Could you check a few things on this model? Use its own coordinates, in mm. Face numbers are marked on the shaded views. A direction names the side the tool comes from. Give positions to 0.01 mm unless a question says otherwise; leave off trailing zeros. Loops run counter-clockwise (first coordinate to the right, second up) from the corner with the lowest first, then second, coordinate; pieces in that order, holes last. Notation, with made-up numbers: (-21, 45.5) -> (-4, 45.5) arc R19 ccw to (-4, 55.5) -> close; hole circle Ø7 at (-12.75, 16). An arc over 180 degrees is marked (long way). Put each result on its own line as item: value.
Autodesk Inventor part; units mm, degrees
ref_plane "YZ Plane" through (0, 0, 0) normal (1, 0, 0) x (0, 1, 0)
ref_plane "XZ Plane" through (0, 0, 0) normal (0, 1, 0) x (-1, 0, 0)
ref_plane "XY Plane" through (0, 0, 0) normal (0, 0, 1) x (1, 0, 0)
sketch "Sketch2" plane through (0, 0, 0) normal (0, 1, 0) x (-1, 0, 0)
  line L0 (18.3186, 20.469) -> (-22.6814, 20.469)
  line L1 (-22.6814, 20.469) -> (-22.6814, -20.531)
  line L2 (-22.6814, -20.531) -> (18.3186, -20.531)
  line L3 (18.3186, -20.531) -> (18.3186, 20.469)
  line L4 (-27.6814, 25.469) -> (23.3186, 25.469)
  line L5 (23.3186, 25.469) -> (23.3186, -25.531)
  line L6 (23.3186, -25.531) -> (-27.6814, -25.531)
  line L7 (-27.6814, -25.531) -> (-27.6814, 25.469)
  line L8 (-22.6814, 20.469) -> (18.3186, 20.469)
  line L9 (18.3186, 20.469) -> (18.3186, -20.531)
  line L10 (18.3186, -20.531) -> (-22.6814, -20.531)
  line L11 (-22.6814, -20.531) -> (-22.6814, 20.469)
  line L12 (-22.6814, 20.469) -> (18.3186, 20.469)
  line L13 (18.3186, 20.469) -> (18.3186, -20.531)
  line L14 (18.3186, -20.531) -> (-22.6814, -20.531)
  line L15 (-22.6814, -20.531) -> (-22.6814, 20.469)
  point P0 (0, 0)
  dimension "d0" = 41
  dimension "d1" = 41
  dimension "d6" = 5
extrude "Extrusion1" add sketch "Sketch2" along normal blind 10 contours L3 L2 L1 L0 | L4 L5 L6 L7
sketch "Sketch5" plane through (0, 0, 0) normal (0, -1, 0) x (1, 0, 0)
  line L0 (27.6814, 25.469) -> (-23.3186, 25.469)
  line L1 (-23.3186, 25.469) -> (-23.3186, -25.531)
  line L2 (-23.3186, -25.531) -> (27.6814, -25.531)
  line L3 (27.6814, -25.531) -> (27.6814, 25.469)
  line L4 (-18.3186, 20.469) -> (22.6814, 20.469)
  line L5 (22.6814, 20.469) -> (22.6814, -20.531)
  line L6 (22.6814, -20.531) -> (-18.3186, -20.531)
  line L7 (-18.3186, -20.531) -> (-18.3186, 20.469)
  point P0 (0, 0)
  dimension "d10" = 5
extrude "Extrusion2" cut sketch "Sketch5" against normal blind 4 contours L4 L5 L6 L7
fillet "Fillet1" radius 3 4 edges at (-23.3186, 10, -0.031) (2.1814, 10, 25.469) (27.6814, 10, -0.031) (2.1814, 10, -25.531)
sketch "Sketch6" plane through (0, 10, 0) normal (0, 1, 0) x (1, 0, 0)
  circle A0 centre (2.1814, 0.031) radius 7.5
  line L0 (-23.3186, 25.531) -> (27.6814, 25.531)
  line L1 (27.6814, -25.469) -> (-23.3186, -25.469)
  point P0 (0, 0)
  dimension "d14" = 15
extrude "Extrusion3" add sketch "Sketch6" along normal blind 50
sketch "Sketch7" plane through (2.1814, 60, -0.031) normal (0, 1, 0) x (1, 0, 0)
  circle A0 centre (0, 0) radius 12.5
  point P0 (-2.1814, -0.031)
  dimension "d17" = 25
extrude "Extrusion4" add sketch "Sketch7" against normal blind 30
fillet "Fillet2" radius 6 1 edges at (-10.3186, 60, -0.031)
fillet "Fillet3" radius 6 1 edges at (-10.3186, 30, -0.031)
fillet "Fillet4" radius 6 1 edges at (-5.3186, 30, -0.031)
fillet "Fillet5" radius 6 1 edges at (-5.3186, 10, -0.031)
properties part number "SMI Stamp Holder"
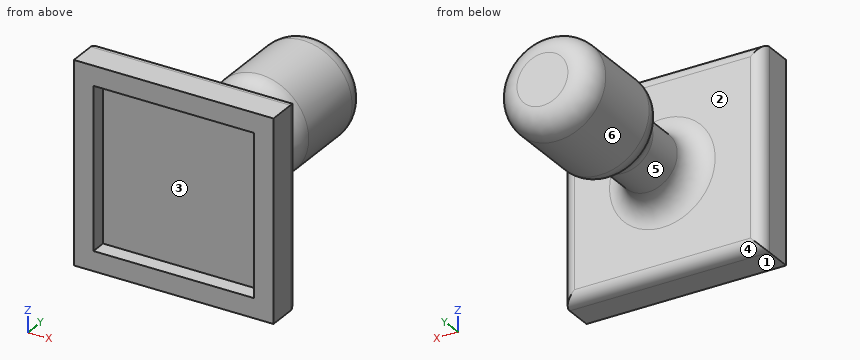
1. If we section it at D-D (y = 32): List the corners of the cut face in (x, z) for me, then the cut area to 3 significant figures.
Recorded:
outline: circle Ø22.09 at (2.18, -0.03)
area: 383 mm^2
2. I need wall thicknesses on line 1 (Y direction, x = 3, z = 16.5); line 2 (Y direction, x = -1, z = -1); line 3 (X direction, y = 3.5, z = -13.5). Which ranges of each line are inside material? Lowest first, please.
Recorded:
line 1: y = 4 to 10
line 2: y = 4 to 60
line 3: x = -23.32 to -18.32, 22.68 to 27.68
3. For the marked faces 1 and 2, which set-ups out of +Z, -Z, +X, -X, +Y, -Y let a thin tool reach every point of the face, with its end or its side?
Recorded:
face 1: -Z, +X, -X, +Y, -Y
face 2: +Y
4. If we section it at C-C (y = 45.5): List the corners of the cut face in (x, z) for me, then the cut area to 3 significant figures.
Recorded:
outline: circle Ø25 at (2.18, -0.03)
area: 491 mm^2
5. Thinking about a two-plate mould opening in Y: for the marked faces 3, 4, 5 and 6, which applies, pulls with the +Y half, pulls with the -Y half, needs draft (parallel to the pull), parting line crosses it, or undercut?
Recorded:
face 3: pulls with the -Y half
face 4: pulls with the +Y half
face 5: undercut
face 6: needs draft
6. If we section it at A-A (x = -17): List the corners of the cut face in (y, z) for me, then the cut area to 3 significant figures.
Recorded:
outline: (0, -25.53) -> (7, -25.53) arc R3 ccw to (10, -22.53) -> (10, 22.47) arc R3 ccw to (7, 25.47) -> (0, 25.47) -> (0, 20.47) -> (4, 20.47) -> (4, -20.53) -> (0, -20.53) -> close
area: 342 mm^2
7. If we section it at B-B (z = -19): List the corners of the cut face in (x, y) for me.
Recorded:
outline: (-23.32, 0) -> (-18.32, 0) -> (-18.32, 4) -> (22.68, 4) -> (22.68, 0) -> (27.68, 0) -> (27.68, 7) arc R3 ccw to (24.68, 10) -> (-20.32, 10) arc R3 ccw to (-23.32, 7) -> close
8. I'm going to push flat-ended pins straight in: pin 1 (12.5 mm diameter, centred on x = 10.5, z = -6.5, fed in from -Y); pin 2 (2 mm diameter, centred on x = 16, y = 36.5, fed in from +Z); pin 3 (10 mm diameter, centred on x = 3, y = 21.5, fed in from -Z); pin 4 (6 mm diameter, centred on y = 23.5, z = -4.5, fed in from +X). Where does each tip first touch, or does it pass through?
Recorded:
pin 1: stops at y = 4
pin 2: passes through
pin 3: stops at z = -7.54
pin 4: stops at x = 9.54
